Can you work these out from the model? Positions are in its coordinate system, mm. A direction names the side the tool comes from. Coordinates: 2 decimals unless noted, no trailing zeros. Order: outer loops, then holes, each group sorted by start corner. A loop starts at its lowest first (then second) coordinate and runs counter-clockwise, first axis right, second up. Notation, with made-up numbers: (61.5, -26) - (66.5, -26) arc R13 ccw to (66.5, -9) - close; hole circle Ø2 at (83, -5.75). An arc over 180 degrees is marked (long way). Return JSON: item names as keys, results as strings. Group by question number.
1) Which directions (+Z, -Z, +X, -X, +Y, -Y) give clear straight access to the entire face, cutting with the end or side of a thin tool? Please do faces 4 (the face through (-12.27, 0.04, 2.67)), 5 (the face through (-12.4, 3, 2.4)), 6 (the face through (-9, -9, 3.75)).
2) For pin 1 Ø1 at (x, y) = (9.5, 5.5) entering from +Z; pin 2 Ø1.1 at (y, z) = (12.5, 1.5) entering from +X; pin 3 Ø1.1 at (y, z) = (-13, 2) entering from -X; pin 4 Ø1.5 at (x, z) = (12.5, 1.5) entering from +Y, each with a flat end and sliding along its axis, tell me the tip position at first contact or that it passes through.
3) Imagine slicing it at C-C (z = 17.25). Write out the boundary of the cut face in (x, y).
4) Imagine slicing it at A-A (y = 0). Give the number of separate pieces and of enclosed holes in the cut face, and give its area (3 significant figures).
5) If we mould it in two halves opening along Y, with no side actions, what happens to faces 1 (the face through (-0.867, -3.905, 9.38)), 2 (the face through (12.4, -4.1, 5)), 3 (the face through (12.3, 3, 2.8))? For each: pulls with the +Y half, pulls with the -Y half, needs draft (parallel to the pull), parting line crosses it, or undercut.
6) If I drill on line 1 along Z through (x, y) = (-9.75, -9.25); line 2 along Z through (x, y) = (-3, 10); line 3 along Y through (x, z) = (10, 0.9), over which ranges is the centre line in solid material (lowest first)?
```python
from build123d import *

# Parameters (mm, degrees)
SKETCH1_R           = 14
BOSS_EXTRUDE1_DEPTH = 18.5
SKETCH2_R           = 14
SKETCH2_R_2         = 5
CUT_EXTRUDE1_DEPTH  = 13.5
SKETCH3_R           = 4
CUT_EXTRUDE2_DEPTH  = 22.5
CUT_EXTRUDE3_DEPTH  = 3.75
SKETCH8_R           = 12.271364757
SKETCH8_R_2         = 6.141449245
CUT_EXTRUDE4_DEPTH  = 2.75
CIRPATTERN1_COUNT   = 4
SKETCH11_R          = 1.5
CUT_EXTRUDE5_DEPTH  = 3


with BuildPart() as part:
    # Sketch1 → Boss-Extrude1 (new body)
    with BuildSketch(Plane.XY):
        Circle(SKETCH1_R)
    extrude(amount=BOSS_EXTRUDE1_DEPTH)

    # Sketch2 → Cut-Extrude1 (cut)
    with BuildSketch(Plane.XY.offset(18.5)):
        Circle(SKETCH2_R)
        Circle(SKETCH2_R_2, mode=Mode.SUBTRACT)
    extrude(amount=-CUT_EXTRUDE1_DEPTH, mode=Mode.SUBTRACT)

    # Sketch3 → Cut-Extrude2 (cut)
    with BuildSketch(Plane.XY.offset(18.5)):
        Circle(SKETCH3_R)
    extrude(amount=-CUT_EXTRUDE2_DEPTH, mode=Mode.SUBTRACT)

    # Sketch6 → Cut-Revolve1 (revolve, cut)
    with BuildSketch(Plane(origin=(0, 0, 0), x_dir=(0, 0, -1), z_dir=(1, 0, 0))):
        Polygon((-4.949121361, 14), (3.777639186, 16.199586118), (5.061522468, 10.233304984), align=None)
    revolve(axis=Axis((0, 0, 19.921792725), (0, 0, -1)), mode=Mode.SUBTRACT)

    # Sketch7 → Cut-Extrude3 (cut)
    with BuildSketch(Plane(origin=(0, 0, 0), x_dir=(-1, 0, 0), z_dir=(0, 0, -1))):
        with BuildLine():
            Line((3, 15.639460569), (3, 11.87697352))
            add(Edge.make_bspline(
                [(3, 11.87697352), (3.121054504, 3.206614769), (11.87697352, 3)],
                knots=[0, 0, 0, 1, 1, 1], degree=2))
            Line((11.87697352, 3), (17.86108213, 3))
            Line((17.86108213, 3), (14.869027825, 14.316513241))
            Line((14.869027825, 14.316513241), (3, 15.639460569))
        make_face()
    cut_extrude3 = extrude(amount=-CUT_EXTRUDE3_DEPTH, mode=Mode.SUBTRACT)

    # Sketch8 → Cut-Extrude4 (cut)
    with BuildSketch(Plane.XY.offset(5)):
        Circle(SKETCH8_R)
        Circle(SKETCH8_R_2, mode=Mode.SUBTRACT)
    extrude(amount=-CUT_EXTRUDE4_DEPTH, mode=Mode.SUBTRACT)

    # Sketch9 → Cut-Revolve2 (revolve, cut)
    with BuildSketch(Plane(origin=(0, 0, 0), x_dir=(1, 0, 0), z_dir=(0, 1, 0))):
        Polygon((-12.001476603, -2.22152714), (-13.001507243, -5.36905248), (-11.155114973, -5.36905248), align=None)
    revolve(axis=Axis((0, 0, -1.742471472), (0, 0, 1)), mode=Mode.SUBTRACT)

    # Sketch10 → Cut-Revolve3 (revolve, cut)
    with BuildSketch(Plane(origin=(0, 0, 0), x_dir=(1, 0, 0), z_dir=(0, 1, 0))):
        Polygon((-5, -5), (-6.141449245, -2.28305418), (-6.572257958, -5.413209842), align=None)
    revolve(axis=Axis((0, 0, 0), (0, 0, -1)), mode=Mode.SUBTRACT)

    # CirPattern1: Cut-Extrude3 ×4 about axis
    cirpattern1_axis = Axis((0, 0, 3.75), (0, 0, 1))
    for i in range(1, CIRPATTERN1_COUNT):
        add(cut_extrude3.rotate(cirpattern1_axis, i * 360 / CIRPATTERN1_COUNT), mode=Mode.SUBTRACT)

    # Sketch11 → Cut-Extrude5 (cut)
    with BuildSketch(Plane(origin=(0, 0, 0), x_dir=(-1, 0, 0), z_dir=(0, 0, -1))):
        with Locations((0, 8)):
            Circle(SKETCH11_R)
        with Locations((0, -8)):
            Circle(SKETCH11_R)
        with Locations((-10, 0)):
            Circle(SKETCH11_R)
        with Locations((10, 0)):
            Circle(SKETCH11_R)
    extrude(amount=-CUT_EXTRUDE5_DEPTH, mode=Mode.SUBTRACT)


solid = part.part
```
Calculated:
{
 "1": {"face 4": "+Z", "face 5": "-Z, -X, +Y", "face 6": "-Z, -X, -Y"},
 "2": {"pin 1": "through", "pin 2": "x = 3", "pin 3": "x = -3", "pin 4": "y = 3"},
 "3": {"outline": "circle Ø10 at (0, 0); hole circle Ø8 at (0, 0)"},
 "4": {"separate pieces": "4", "enclosed holes": "0", "area": "66.3 mm2"},
 "5": {"face 1": "undercut", "face 2": "needs draft", "face 3": "pulls with the +Y half"},
 "6": {"line 1": "3.75 to 5", "line 2": "0 to 2.25", "line 3": "-3.16 to -1.5, 1.5 to 3.14"}
}
